Work out the finished part from the listing and answer in its coordinate system (mm). A direction names the side the tool comes from. Give positions to 0.01 mm unless a question says otherwise; leave off trailing zeros. Loops run counter-clockwise (first coordinate to the right, second up) from the corner with the lowest first, then second, coordinate; pieces in that order, holes last. Notation, with made-up numbers: (-23, 24.5) - (30, 24.5) arc R17 ccw to (30, 38.5) - close; hole circle Ø10 at (38.5, 18). An arc over 180 degrees is marked (long way). Use CSV: the item, a comma, the result in double quotes.
from build123d import *

# Parameters (mm, degrees)
CYLINDER001_R     = 3.5
CYLINDER001_DEPTH = 10
CYLINDER002_R     = 1.5
CYLINDER002_DEPTH = 7.5
CYLINDER003_R     = 3.5
CYLINDER003_DEPTH = 10
CYLINDER_R        = 1.5
CYLINDER_DEPTH    = 7.5
EXTRUDE_DEPTH     = 15
CHAMFER_SIZE      = 2


with BuildPart() as screwheadhole000:
    # Cylinder001 → Cylinder001 (new body)
    with BuildSketch(Plane(origin=(12.5, 17.5, 7.5), x_dir=(1, 0, 0), z_dir=(0, -1, 0))):
        Circle(CYLINDER001_R)
    extrude(amount=CYLINDER001_DEPTH)


with BuildPart() as screwhole001:
    # Cylinder002 → Cylinder002 (new body)
    with BuildSketch(Plane(origin=(162.5, 7.5, 7.5), x_dir=(1, 0, 0), z_dir=(0, -1, 0))):
        Circle(CYLINDER002_R)
    extrude(amount=CYLINDER002_DEPTH)


with BuildPart() as screwheadhole001:
    # Cylinder003 → Cylinder003 (new body)
    with BuildSketch(Plane(origin=(162.5, 17.5, 7.5), x_dir=(1, 0, 0), z_dir=(0, -1, 0))):
        Circle(CYLINDER003_R)
    extrude(amount=CYLINDER003_DEPTH)


with BuildPart() as fusion:
    # Cylinder → Cylinder (new body)
    with BuildSketch(Plane(origin=(12.5, 7.5, 7.5), x_dir=(1, 0, 0), z_dir=(0, -1, 0))):
        Circle(CYLINDER_R)
    extrude(amount=CYLINDER_DEPTH)

    # Fusion: union screwheadhole000, screwhole001, screwheadhole001
    add(screwheadhole000.part)
    add(screwhole001.part)
    add(screwheadhole001.part)


with BuildPart() as cut:
    # Sketch → Extrude (new body)
    with BuildSketch(Plane.XY):
        Polygon((0, 0), (25, 0), (25, 10), (30, 15), (145, 15), (150, 10), (150, 0), (175, 0), (150, 25), (25, 25), align=None)
    extrude(amount=EXTRUDE_DEPTH)

    # Chamfer
    chamfer_edges = [cut.edges().sort_by_distance(p)[0] for p in [
        (25, 5, 0),
        (25, 5, 15),
        (27.5, 12.5, 0),
        (27.5, 12.5, 15),
        (87.5, 15, 0),
        (87.5, 15, 15),
        (147.5, 12.5, 0),
        (147.5, 12.5, 15),
        (150, 5, 0),
        (150, 5, 15),
        (162.5, 12.5, 0),
        (162.5, 12.5, 15),
        (87.5, 25, 0),
        (87.5, 25, 15),
        (12.5, 12.5, 0),
        (12.5, 12.5, 15),
    ]]
    chamfer(chamfer_edges, length=CHAMFER_SIZE)

    # Cut: cut Fusion
    add(fusion.part, mode=Mode.SUBTRACT)


solid = cut.part
Item 1: Given P1, Ø3, axis at y = 18.5, z = 8.5, coming from the -X side; P2, Ø9, axis at x = 162.5, z = 7.5, coming from the +Y side; P3, Ø9, axis at x = 99, z = 6.5, coming from the -Y side, each flat-ended and moving along its own axis, determine where each tip first touches the part or whether it passes through.
Determined:
P1,"stops at x = 17"
P2,"stops at y = 17"
P3,"stops at y = 15"
Item 2: For faces 4 (the flat face through (163.2, 7.5, 6)), 5 (the flat face through (148.17, 13.26, 0.99)), 6 (the flat face through (27, 12, 7)), 7 (the flat face through (87, 18, 0)), 8 (the flat face through (87, 18, 15)), determine the directions among +Z, -Z, +X, -X, +Y, -Y from which every point of the face is accessible in a straight line to the end or side of a thin tool.
Determined:
face 4,"+Y"
face 5,"-Z, -Y"
face 6,"+Z, -Z, -Y"
face 7,"-Z, +X, -X, +Y, -Y"
face 8,"+Z, +X, -X, +Y, -Y"
Item 3: The mould has two halves that part along X. Classify faces 1 (the flat face through (88, 25, 7)), 2 (the flat face through (25, 5, 7)), 3 (the flat face through (161.96, 11.61, 0.99)): pulls with the +X half, pulls with the -X half, needs draft (parallel to the pull), parting line crosses it, or undercut.
Determined:
face 1,"needs draft"
face 2,"undercut"
face 3,"pulls with the +X half"
Item 4: Find the intervals of material crossed by line 1 (Y direction, x = 63.5, z = 5.75); line 2 (X direction, y = 8.25, z = 3.25); line 3 (X direction, y = 2.5, z = 2.5), in increasing order.
Determined:
line 1,"y = 15 to 25"
line 2,"x = 8.25 to 25, 150 to 166.75"
line 3,"x = 2.5 to 25, 150 to 172.5"
Item 5: A cutting plane is placed at B-B on y = 3.25. Determine the outline of the cut face in (x, z).
Determined:
outline,"(3.25, 2) - (6.08, 0) - (23, 0) - (25, 2) - (25, 13) - (23, 15) - (6.08, 15) - (3.25, 13) - close; (150, 2) - (152, 0) - (168.92, 0) - (171.75, 2) - (171.75, 13) - (168.92, 15) - (152, 15) - (150, 13) - close; hole circle Ø3 at (12.5, 7.5); hole circle Ø3 at (162.5, 7.5)"
Item 6: A cutting plane is placed at A-A on z = 7.5. Determine the outline of the cut face in (x, y).
Determined:
outline,"(0, 0) - (11, 0) - (11, 7.5) - (9, 7.5) - (9, 9) - close; (14, 0) - (25, 0) - (25, 10) - (30, 15) - (145, 15) - (150, 10) - (150, 0) - (161, 0) - (161, 7.5) - (159, 7.5) - (159, 16) - (150, 25) - (25, 25) - (16, 16) - (16, 7.5) - (14, 7.5) - close; (164, 0) - (175, 0) - (166, 9) - (166, 7.5) - (164, 7.5) - close"
Item 7: A cutting plane is placed at C-C on x = 12.5. Determine the outline of the cut face in (y, z), and give its area (3 significant figures).
Determined:
outline,"(0, 0) - (9.67, 0) - (12.5, 2) - (12.5, 4) - (7.5, 4) - (7.5, 6) - (0, 6) - close; (0, 9) - (7.5, 9) - (7.5, 11) - (12.5, 11) - (12.5, 13) - (9.67, 15) - (0, 15) - close"
area,"124 mm²"
Item 8: A cutting plane is placed at D-D on x = 94. Determine the outline of the cut face in (y, z).
Determined:
outline,"(15, 2) - (17, 0) - (23, 0) - (25, 2) - (25, 13) - (23, 15) - (17, 15) - (15, 13) - close"
